Check sheet for the modelled part. Datum: model origin and axes. Units: mm. Give positions to 0.01 mm unless a question says otherwise; leave off trailing zeros. Loops run counter-clockwise (first coordinate to the right, second up) from the corner with the lowest first, then second, coordinate; pieces in that order, holes last. Notation, with made-up numbers: M 49,69.5 L 95,69.5 A21 ccw 95,81.5 Z; hole C 89.25,-25.5 d10. An arc over 180 degrees is marked long. Write each question's results on one line, items separated by ' | '. Start each with the question number.
1. Sectioned sample at A-A on y = -25. Record the cut outline in (x, z).
2. Material ranges on line 1 along Y through (x, z) = (57, 1.8); line 2 along Y through (x, z) = (-26, 3.9); line 3 along Y through (x, z) = (-42, 1.15), recorded low to high.
3. Sectioned sample at D-D on x = 10. Record the cut outline in (y, z).
4. Sectioned sample at C-C on y = -7.5. Record the cut outline in (x, z), and give its area (3 significant figures).
5. Go/stop test with flat-tipped pins: pin 1 (2 mm diameter, centred on x = -44.5, z = 3, fed in from +Y); pin 2 (1.5 mm diameter, centred on x = -0.5, z = 1.5, fed in from +Y); pin 3 (1.3 mm diameter, centred on y = -13, z = 3, fed in from -X). Record where each tip stops, or that it passes through.
6. Sectioned sample at B-B on x = -25. Record the cut outline in (y, z), and give its area (4 significant figures).
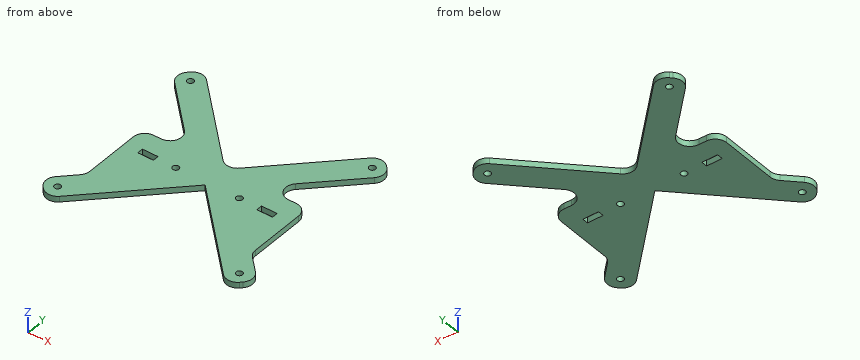
```python
from build123d import *

# Parameters (mm, degrees)
BOSS_EXTRUDE1_DEPTH     = 4.5
SKETCH3_R               = 2.5
CUT_EXTRUDE3_DEPTH      = 118.194127679
FILLET1_R               = 9
FILLET2_R               = 9
SKETCH5_R               = 2.5
CUT_EXTRUDE4_DEPTH      = 112.927846314
MIRROR2_COPY_1_SKETCH_R = 2.5
MIRROR2_COPY_1_DEPTH    = 112.927846314


with BuildPart() as part:
    # Sketch1 → Boss-Extrude1 (new body)
    with BuildSketch(Plane.XY):
        Polygon((-28.284271247, -10), (-6.15, -10), (-6.15, -5.3), (6.15, -5.3), (6.15, -10), (28.284271247, -10), (40.65, -10), (40.65, -5.3), (52.95, -5.3), (52.95, -10), (65, -10), (65, 10), (28.284271247, 10), (0, 10), (-28.284271247, 10), (-65, 10), (-65, -10), (-52.95, -10), (-52.95, -5.3), (-40.65, -5.3), (-40.65, -10), align=None)
        Polygon((-70.710678119, -80.710678119), (0, -10), (-6.15, -10), (-28.284271247, -10), (-65, -46.715728753), (-84.852813742, -66.568542495), align=None)
        Polygon((6.15, -10), (0, -10), (70.710678119, -80.710678119), (84.852813742, -66.568542495), (65, -46.715728753), (28.284271247, -10), align=None)
        Polygon((0, 10), (28.284271247, 10), (84.852813742, 66.568542495), (70.710678119, 80.710678119), align=None)
        Polygon((-84.852813742, 66.568542495), (-28.284271247, 10), (0, 10), (-70.710678119, 80.710678119), align=None)
        Polygon((-6.15, -10), (0, -10), (6.15, -10), (6.15, -5.3), (-6.15, -5.3), align=None)
        Polygon((-65, -46.715728753), (-28.284271247, -10), (-40.65, -10), (-52.95, -10), (-65, -10), align=None)
        Polygon((40.65, -10), (28.284271247, -10), (65, -46.715728753), (65, -10), (52.95, -10), align=None)
    extrude(amount=BOSS_EXTRUDE1_DEPTH)

    # Sketch3 → Cut-Extrude3 (cut, through all)
    with BuildSketch(Plane.XY.offset(4.5)):
        with Locations((-25, -7.5)):
            Circle(SKETCH3_R)
        with Locations((25, -7.5)):
            Circle(SKETCH3_R)
    extrude(amount=-CUT_EXTRUDE3_DEPTH, mode=Mode.SUBTRACT)

    # Fillet1
    fillet1_edges = [part.edges().sort_by_distance(p)[0] for p in [
        (-65, -46.715728753, 2.25),
        (-65, 10, 2.25),
        (-28.284271247, 10, 2.25),
        (0, 10, 2.25),
        (28.284271247, 10, 2.25),
        (65, 10, 2.25),
        (65, -46.715728753, 2.25),
    ]]
    fillet(fillet1_edges, radius=FILLET1_R)

    # Fillet2
    fillet2_edges = [part.edges().sort_by_distance(p)[0] for p in [
        (-70.710678119, -80.710678119, 2.25),
        (-84.852813742, -66.568542495, 2.25),
        (-84.852813742, 66.568542495, 2.25),
        (-70.710678119, 80.710678119, 2.25),
        (70.710678119, 80.710678119, 2.25),
        (84.852813742, 66.568542495, 2.25),
        (84.852813742, -66.568542495, 2.25),
        (70.710678119, -80.710678119, 2.25),
    ]]
    fillet(fillet2_edges, radius=FILLET2_R)

    # Sketch5 → Cut-Extrude4 (cut, through all)
    with BuildSketch(Plane.XY.offset(4.5)):
        with Locations((-71.4177849, 67.275649276)):
            Circle(SKETCH5_R)
    cut_extrude4 = extrude(amount=-CUT_EXTRUDE4_DEPTH, mode=Mode.SUBTRACT)

    # Mirror1: Cut-Extrude4 across plane
    add(cut_extrude4.mirror(Plane(origin=(0, 0, 0), x_dir=(0, 0, 1), z_dir=(1, 0, 0))), mode=Mode.SUBTRACT)

    # Mirror2: Cut-Extrude4 across plane
    add(cut_extrude4.mirror(Plane.ZX), mode=Mode.SUBTRACT)

    # Mirror2 copy 1 sketch → Mirror2 copy 1 (cut, through all)
    with BuildSketch(Plane(origin=(0, 0, 4.5), x_dir=(-1, 0, 0), z_dir=(0, 0, 1))):
        with Locations((-71.4177849, 67.275649276)):
            Circle(MIRROR2_COPY_1_SKETCH_R)
    extrude(amount=-MIRROR2_COPY_1_DEPTH, mode=Mode.SUBTRACT)


solid = part.part
```
Output values:
1) outline: M -65,0 L -15,0 L -15,4.5 L -65,4.5 Z; M 15,0 L 65,0 L 65,4.5 L 15,4.5 Z
2) line 1: -67 to 9.94, 38.72 to 67 | line 2: -36 to -9.79, -5.21 to 36 | line 3: -52 to -10, -5.3 to 14.9, 23.1 to 52
3) outline: M -20,0 L 20,0 L 20,4.5 L -20,4.5 Z
4) outline: M -65,0 L -52.95,0 L -52.95,4.5 L -65,4.5 Z; M -40.65,0 L -27.5,0 L -27.5,4.5 L -40.65,4.5 Z; M -22.5,0 L 22.5,0 L 22.5,4.5 L -22.5,4.5 Z; M 27.5,0 L 40.65,0 L 40.65,4.5 L 27.5,4.5 Z; M 52.95,0 L 65,0 L 65,4.5 L 52.95,4.5 Z | area: 429 mm2
5) pin 1: y = 55.5 | pin 2: y = 13.82 | pin 3: x = -65
6) outline: M -35,0 L -10,0 L -10,4.5 L -35,4.5 Z; M -5,0 L 35,0 L 35,4.5 L -5,4.5 Z | area: 292.5 mm2
